Source: CAD feature listing. Evaluate the final solid. Frame: model axes, mm. Face numbers are marked on the shaded views. Coordinates: 2 decimals unless noted, no trailing zeros. Write each loop counter-clockwise with the first axis right and the second up, starting at its lowest first coordinate (ties: lowest second). Pieces come first, ordered by that corner, then holes. Notation, with made-up numbers: (62.5, 78.5) -> (118.5, 78.5) arc R21 ccw to (118.5, 92.5) -> close; hole circle Ø11 at (-28, 66). An arc over 180 degrees is marked (long way). One line per item, written item: value. Start each with the question number.
1. Line query: line 1 (X direction, y = 1, z = 58.5); line 2 (Y direction, x = 35.5, z = 45.5); line 3 (X direction, y = 15.25, z = 23.5). Output: solid intervals per line, ascending.
2. Mould query, pull axis Y, two halves, no side actions, for the marked faces 1, 2 and 3. Classes: released by +Y, released by -Y, zero draft, split by the parting line, or undercut.
3. Section query A-A, the plane y = 10. Output: boundary loops of the cut face in (x, z).
4. Section query C-C, the plane y = 15. Output: boundary loops of the cut face in (x, z).
5. Section query B-B, the plane x = 19.5. Output: boundary loops of the cut face in (y, z), and give its area (3 significant figures).
6. First-contact query: P1, Ø0.6, axis at x = 33.5, z = 48, coming from the +Y side; P2, Ø0.6, axis at x = 26.5, z = 38, coming from the -Y side. Flat tips, straight axial feed; report the tip coordinate or a pass-through.
7. Section query D-D, the plane z = 65. State how many separate pieces and enclosed holes the cut face has, and give its area (3 significant figures).
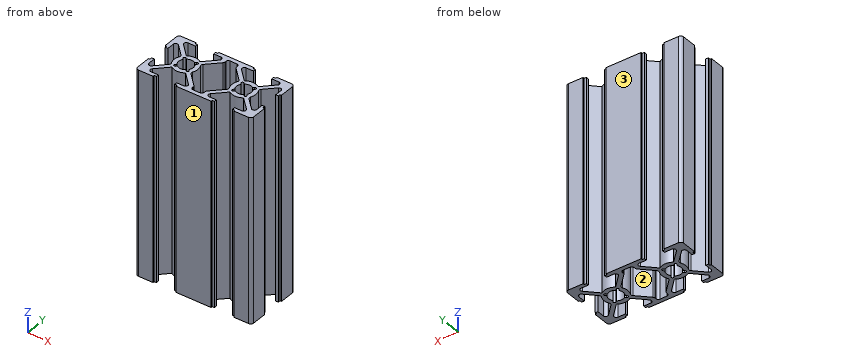
from build123d import *

# Parameters (mm, degrees)
Y_KSEKLIK_EKSTR_ZYON2_DEPTH = 70
RADYUS1_R                   = 0.8


with BuildPart() as part:
    # Çizim3 → Yükseklik-Ekstrüzyon2 (new body)
    with BuildSketch(Plane.XY):
        with BuildLine():
            Line((1, 0), (6.1, 0))
            Line((6.1, 0), (6.1, 0.5))
            Line((6.1, 0.5), (6.85, 0.5))
            Line((6.85, 0.5), (6.85, 1.4))
            Line((6.85, 1.4), (4.321320344, 1.4))
            ThreePointArc((4.321320344, 1.4), (3.582216718, 1.893853254), (3.755634919, 2.765685425))
            Line((3.755634919, 2.765685425), (7.638403375, 6.648453882))
            ThreePointArc((7.638403375, 6.648453882), (10, 5.9), (12.361596625, 6.648453882))
            Line((12.361596625, 6.648453882), (16.244365081, 2.765685425))
            ThreePointArc((16.244365081, 2.765685425), (16.417783282, 1.893853254), (15.678679656, 1.4))
            Line((15.678679656, 1.4), (13.15, 1.4))
            Line((13.15, 1.4), (13.15, 0.5))
            Line((13.15, 0.5), (13.9, 0.5))
            Line((13.9, 0.5), (13.9, 0))
            Line((13.9, 0), (26.1, 0))
            Line((26.1, 0), (26.1, 0.5))
            Line((26.1, 0.5), (26.85, 0.5))
            Line((26.85, 0.5), (26.85, 1.4))
            Line((26.85, 1.4), (24.321320344, 1.4))
            ThreePointArc((24.321320344, 1.4), (23.582216718, 1.893853254), (23.755634919, 2.765685425))
            Line((23.755634919, 2.765685425), (27.638403375, 6.648453882))
            ThreePointArc((27.638403375, 6.648453882), (30, 5.9), (32.361596625, 6.648453882))
            Line((32.361596625, 6.648453882), (36.244365081, 2.765685425))
            ThreePointArc((36.244365081, 2.765685425), (36.417783282, 1.893853254), (35.678679656, 1.4))
            Line((35.678679656, 1.4), (33.15, 1.4))
            Line((33.15, 1.4), (33.15, 0.5))
            Line((33.15, 0.5), (33.9, 0.5))
            Line((33.9, 0.5), (33.9, 0))
            Line((33.9, 0), (39, 0))
            ThreePointArc((39, 0), (39.707106781, 0.292893219), (40, 1))
            Line((40, 1), (40, 6.1))
            Line((40, 6.1), (39.5, 6.1))
            Line((39.5, 6.1), (39.5, 6.85))
            Line((39.5, 6.85), (38.6, 6.85))
            Line((38.6, 6.85), (38.6, 4.321320344))
            ThreePointArc((38.6, 4.321320344), (38.106146746, 3.582216718), (37.234314575, 3.755634919))
            Line((37.234314575, 3.755634919), (33.351546118, 7.638403375))
            ThreePointArc((33.351546118, 7.638403375), (34.1, 10), (33.351546118, 12.361596625))
            Line((33.351546118, 12.361596625), (37.234314575, 16.244365081))
            ThreePointArc((37.234314575, 16.244365081), (38.106146746, 16.417783282), (38.6, 15.678679656))
            Line((38.6, 15.678679656), (38.6, 13.15))
            Line((38.6, 13.15), (39.5, 13.15))
            Line((39.5, 13.15), (39.5, 13.9))
            Line((39.5, 13.9), (40, 13.9))
            Line((40, 13.9), (40, 19))
            ThreePointArc((40, 19), (39.707106781, 19.707106781), (39, 20))
            Line((39, 20), (33.9, 20))
            Line((33.9, 20), (33.9, 19.5))
            Line((33.9, 19.5), (33.15, 19.5))
            Line((33.15, 19.5), (33.15, 18.6))
            Line((33.15, 18.6), (35.678679656, 18.6))
            ThreePointArc((35.678679656, 18.6), (36.417783282, 18.106146746), (36.244365081, 17.234314575))
            Line((36.244365081, 17.234314575), (32.361596625, 13.351546118))
            ThreePointArc((32.361596625, 13.351546118), (30, 14.1), (27.638403375, 13.351546118))
            Line((27.638403375, 13.351546118), (23.755634919, 17.234314575))
            ThreePointArc((23.755634919, 17.234314575), (23.582216718, 18.106146746), (24.321320344, 18.6))
            Line((24.321320344, 18.6), (26.85, 18.6))
            Line((26.85, 18.6), (26.85, 19.5))
            Line((26.85, 19.5), (26.1, 19.5))
            Line((26.1, 19.5), (26.1, 20))
            Line((26.1, 20), (13.9, 20))
            Line((13.9, 20), (13.9, 19.5))
            Line((13.9, 19.5), (13.15, 19.5))
            Line((13.15, 19.5), (13.15, 18.6))
            Line((13.15, 18.6), (15.678679656, 18.6))
            ThreePointArc((15.678679656, 18.6), (16.417783282, 18.106146746), (16.244365081, 17.234314575))
            Line((16.244365081, 17.234314575), (12.361596625, 13.351546118))
            ThreePointArc((12.361596625, 13.351546118), (10, 14.1), (7.638403375, 13.351546118))
            Line((7.638403375, 13.351546118), (3.755634919, 17.234314575))
            ThreePointArc((3.755634919, 17.234314575), (3.582216718, 18.106146746), (4.321320344, 18.6))
            Line((4.321320344, 18.6), (6.85, 18.6))
            Line((6.85, 18.6), (6.85, 19.5))
            Line((6.85, 19.5), (6.1, 19.5))
            Line((6.1, 19.5), (6.1, 20))
            Line((6.1, 20), (1, 20))
            ThreePointArc((1, 20), (0.292893219, 19.707106781), (0, 19))
            Line((0, 19), (0, 13.9))
            Line((0, 13.9), (0.5, 13.9))
            Line((0.5, 13.9), (0.5, 13.15))
            Line((0.5, 13.15), (1.4, 13.15))
            Line((1.4, 13.15), (1.4, 15.678679656))
            ThreePointArc((1.4, 15.678679656), (1.893853254, 16.417783282), (2.765685425, 16.244365081))
            Line((2.765685425, 16.244365081), (6.648453882, 12.361596625))
            ThreePointArc((6.648453882, 12.361596625), (5.9, 10), (6.648453882, 7.638403375))
            Line((6.648453882, 7.638403375), (2.765685425, 3.755634919))
            ThreePointArc((2.765685425, 3.755634919), (1.893853254, 3.582216718), (1.4, 4.321320344))
            Line((1.4, 4.321320344), (1.4, 6.85))
            Line((1.4, 6.85), (0.5, 6.85))
            Line((0.5, 6.85), (0.5, 6.1))
            Line((0.5, 6.1), (0, 6.1))
            Line((0, 6.1), (0, 1))
            ThreePointArc((0, 1), (0.292893219, 0.292893219), (1, 0))
        make_face()
        with BuildLine():
            Line((21.210320913, 18.6), (18.789679087, 18.6))
            ThreePointArc((18.789679087, 18.6), (18.223993662, 18.365685425), (17.989679087, 17.8))
            Line((17.989679087, 17.8), (17.989679087, 17.331100443))
            ThreePointArc((17.989679087, 17.331100443), (17.928782713, 17.024953697), (17.755364512, 16.765415018))
            Line((17.755364512, 16.765415018), (13.351546118, 12.361596625))
            ThreePointArc((13.351546118, 12.361596625), (14.1, 10), (13.351546118, 7.638403375))
            Line((13.351546118, 7.638403375), (17.755364512, 3.234584982))
            ThreePointArc((17.755364512, 3.234584982), (17.928782713, 2.975046303), (17.989679087, 2.668899557))
            Line((17.989679087, 2.668899557), (17.989679087, 2.2))
            ThreePointArc((17.989679087, 2.2), (18.223993662, 1.634314575), (18.789679087, 1.4))
            Line((18.789679087, 1.4), (21.210320913, 1.4))
            ThreePointArc((21.210320913, 1.4), (21.776006338, 1.634314575), (22.010320913, 2.2))
            Line((22.010320913, 2.2), (22.010320913, 2.668899557))
            ThreePointArc((22.010320913, 2.668899557), (22.071217287, 2.975046303), (22.244635488, 3.234584982))
            Line((22.244635488, 3.234584982), (26.648453882, 7.638403375))
            ThreePointArc((26.648453882, 7.638403375), (25.9, 10), (26.648453882, 12.361596625))
            Line((26.648453882, 12.361596625), (22.244635488, 16.765415018))
            ThreePointArc((22.244635488, 16.765415018), (22.071217287, 17.024953697), (22.010320913, 17.331100443))
            Line((22.010320913, 17.331100443), (22.010320913, 17.8))
            ThreePointArc((22.010320913, 17.8), (21.776006338, 18.365685425), (21.210320913, 18.6))
        make_face(mode=Mode.SUBTRACT)
        with BuildLine():
            Line((8.201142588, 12.443783276), (8.552743846, 12.092182018))
            ThreePointArc((8.552743846, 12.092182018), (10, 12.543968548), (11.447256154, 12.092182018))
            Line((11.447256154, 12.092182018), (11.798857412, 12.443783276))
            ThreePointArc((11.798857412, 12.443783276), (12.443783276, 12.443783276), (12.443783276, 11.798857412))
            Line((12.443783276, 11.798857412), (12.092182018, 11.447256154))
            ThreePointArc((12.092182018, 11.447256154), (12.543968548, 10), (12.092182018, 8.552743846))
            Line((12.092182018, 8.552743846), (12.443783276, 8.201142588))
            ThreePointArc((12.443783276, 8.201142588), (12.443783276, 7.556216724), (11.798857412, 7.556216724))
            Line((11.798857412, 7.556216724), (11.447256154, 7.907817982))
            ThreePointArc((11.447256154, 7.907817982), (10, 7.456031452), (8.552743846, 7.907817982))
            Line((8.552743846, 7.907817982), (8.201142588, 7.556216724))
            ThreePointArc((8.201142588, 7.556216724), (7.556216724, 7.556216724), (7.556216724, 8.201142588))
            Line((7.556216724, 8.201142588), (7.907817982, 8.552743846))
            ThreePointArc((7.907817982, 8.552743846), (7.456031452, 10), (7.907817982, 11.447256154))
            Line((7.907817982, 11.447256154), (7.556216724, 11.798857412))
            ThreePointArc((7.556216724, 11.798857412), (7.556216724, 12.443783276), (8.201142588, 12.443783276))
        make_face(mode=Mode.SUBTRACT)
        with BuildLine():
            Line((27.907817982, 11.447256154), (27.556216724, 11.798857412))
            ThreePointArc((27.556216724, 11.798857412), (27.556216724, 12.443783276), (28.201142588, 12.443783276))
            Line((28.201142588, 12.443783276), (28.552743846, 12.092182018))
            ThreePointArc((28.552743846, 12.092182018), (30, 12.543968548), (31.447256154, 12.092182018))
            Line((31.447256154, 12.092182018), (31.798857412, 12.443783276))
            ThreePointArc((31.798857412, 12.443783276), (32.443783276, 12.443783276), (32.443783276, 11.798857412))
            Line((32.443783276, 11.798857412), (32.092182018, 11.447256154))
            ThreePointArc((32.092182018, 11.447256154), (32.543968548, 10), (32.092182018, 8.552743846))
            Line((32.092182018, 8.552743846), (32.443783276, 8.201142588))
            ThreePointArc((32.443783276, 8.201142588), (32.443783276, 7.556216724), (31.798857412, 7.556216724))
            Line((31.798857412, 7.556216724), (31.447256154, 7.907817982))
            ThreePointArc((31.447256154, 7.907817982), (30, 7.456031452), (28.552743846, 7.907817982))
            Line((28.552743846, 7.907817982), (28.201142588, 7.556216724))
            ThreePointArc((28.201142588, 7.556216724), (27.556216724, 7.556216724), (27.556216724, 8.201142588))
            Line((27.556216724, 8.201142588), (27.907817982, 8.552743846))
            ThreePointArc((27.907817982, 8.552743846), (27.456031452, 10), (27.907817982, 11.447256154))
        make_face(mode=Mode.SUBTRACT)
    extrude(amount=Y_KSEKLIK_EKSTR_ZYON2_DEPTH)

    # Radyus1
    radyus1_edges = [part.edges().sort_by_distance(p)[0] for p in [
        (6.648453882, 7.638403375, 35),
        (6.648453882, 12.361596625, 35),
        (33.351546118, 12.361596625, 35),
        (33.351546118, 7.638403375, 35),
        (13.351546118, 12.361596625, 35),
        (13.351546118, 7.638403375, 35),
        (26.648453882, 7.638403375, 35),
        (26.648453882, 12.361596625, 35),
    ]]
    fillet(radyus1_edges, radius=RADYUS1_R)


solid = part.part
Computed values:
1. line 1: x = 0 to 6.85, 13.15 to 26.85, 33.15 to 40
1. line 2: y = 0 to 1.4, 3.51 to 5.49, 14.51 to 16.49, 18.6 to 20
1. line 3: x = 0 to 1.4, 3.76 to 5.74, 14.26 to 16.24, 23.76 to 25.74, 34.26 to 36.24, 38.6 to 40
2. face 1: released by -Y
2. face 2: undercut
2. face 3: released by +Y
3. outline: (5.9, 0) -> (7.46, 0) -> (7.46, 70) -> (5.9, 70) -> close; (12.54, 0) -> (14.1, 0) -> (14.1, 70) -> (12.54, 70) -> close; (25.9, 0) -> (27.46, 0) -> (27.46, 70) -> (25.9, 70) -> close; (32.54, 0) -> (34.1, 0) -> (34.1, 70) -> (32.54, 70) -> close
4. outline: (0, 0) -> (1.4, 0) -> (1.4, 70) -> (0, 70) -> close; (4.01, 0) -> (5.99, 0) -> (5.99, 70) -> (4.01, 70) -> close; (14.01, 0) -> (15.99, 0) -> (15.99, 70) -> (14.01, 70) -> close; (24.01, 0) -> (25.99, 0) -> (25.99, 70) -> (24.01, 70) -> close; (34.01, 0) -> (35.99, 0) -> (35.99, 70) -> (34.01, 70) -> close; (38.6, 0) -> (40, 0) -> (40, 70) -> (38.6, 70) -> close
5. outline: (0, 0) -> (1.4, 0) -> (1.4, 70) -> (0, 70) -> close; (18.6, 0) -> (20, 0) -> (20, 70) -> (18.6, 70) -> close
5. area: 196 mm²
6. P1: stops at y = 19.5
6. P2: stops at y = 0.5
7. separate pieces: 1
7. enclosed holes: 3
7. area: 255 mm²
